Could you check a few things on this model? Use its own coordinates, in mm. Give positions to 0.01 mm unless a question says otherwise; leave off trailing zeros. Loops run counter-clockwise (first coordinate to the right, second up) from the corner with the lowest first, then second, coordinate; pieces in that order, holes last. Notation, with made-up numbers: (-29, 67) -> (-9, 67) arc R23 ccw to (-9, 78) -> close; hole circle Ø1 at (45.25, 41.5). An arc over 180 degrees is marked (long way). Write each question's results on one line, items separated by ' | '. Start each with the question number.
Q1. If we section it at A-A, the plane x = 32: List the corners of the cut face in (y, z) for me.
Q2. If we section it at D-D, the plane x = -97.5: List the corners of the cut face in (y, z) for me.
Q3. If we section it at B-B, the plane y = 51: List the corners of the cut face in (x, z) for me, plus the area to 3 significant figures.
Q4. If we section it at C-C, the plane z = 1: Give the number of separate pieces and of enclosed holes in the cut face, plus the area to 3 significant figures.
Q5. If I drill on line 1 along Y through (x, z) = (-14, 1.4); line 2 along X through (y, z) = (64, 0.85); line 3 along X through (y, z) = (10.5, 1.15), over which ranges is the centre line in solid material (lowest first)?
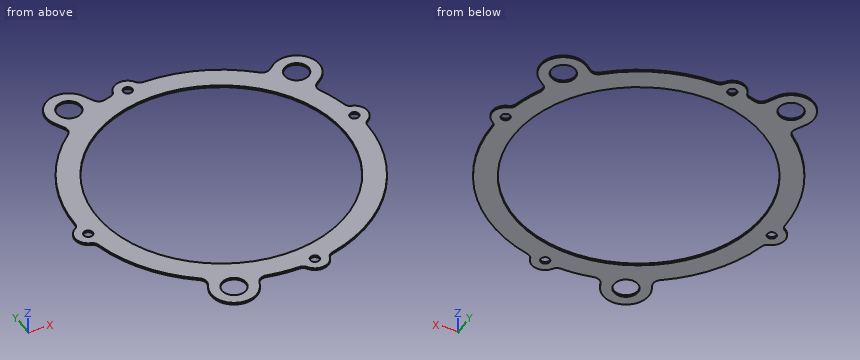
from build123d import *

# Parameters (mm, degrees)
F0_R     = 9
F0_R_2   = 3.4
F0_R_3   = 92.5
F1_DEPTH = 1.5
F2_R     = 6
F3_R     = 5


# Not quite as in the source:
# - a feature names something its author has since deleted; it is built from what else it names


with BuildPart() as f1:
    # F0 (on Top) → F1 (new body)
    with BuildSketch(Plane.XY):
        with BuildLine():
            ThreePointArc((-41.5612142371, 114.3762015069), (-64.5523398831, 121.4052940181), (-71.5814323943, 98.4141683721))
            Line((-71.5814323943, 98.4141683721), (-65.4484708904, 86.8797453608))
            ThreePointArc((-65.4484708904, 86.8797453608), (-98.0871820311, 47.0159251428), (-108.7201014418, -3.3958854983))
            ThreePointArc((-108.7201014418, -3.3958854983), (-115.9027148008, -14.2310639443), (-106.3121888463, -23.0067598447))
            ThreePointArc((-106.3121888463, -23.0067598447), (-89.5246549559, -61.7812969341), (-59.2286170286, -91.2335652089))
            Line((-59.2286170286, -91.2335652089), (-62.9150916983, -99.5135228831))
            ThreePointArc((-62.9150916983, -99.5135228831), (-54.2993418506, -121.9583185953), (-31.8545461384, -113.3425687477))
            Line((-31.8545461384, -113.3425687477), (-28.1680714687, -105.0626110734))
            ThreePointArc((-28.1680714687, -105.0626110734), (-12.5203677417, -108.0501406174), (3.3958854983, -108.7201014418))
            ThreePointArc((3.3958854983, -108.7201014418), (14.2310639443, -115.9027148008), (23.0067598447, -106.3121888463))
            ThreePointArc((23.0067598447, -106.3121888463), (85.7143913832, -66.9674219725), (108.7201014418, 3.3958854983))
            ThreePointArc((108.7201014418, 3.3958854983), (115.9027148008, 14.2310639443), (106.3121888463, 23.0067598447))
            ThreePointArc((106.3121888463, 23.0067598447), (102.1418848281, 37.3982333755), (96.0334257824, 51.0800707549))
            Line((96.0334257824, 51.0800707549), (104.0705278241, 57.1364615496))
            ThreePointArc((104.0705278241, 57.1364615496), (107.4164761014, 80.944120614), (83.608817037, 84.2900688912))
            Line((83.608817037, 84.2900688912), (75.5717149953, 78.2336780965))
            ThreePointArc((75.5717149953, 78.2336780965), (39.1751591317, 101.4736389554), (-3.3958854983, 108.7201014418))
            ThreePointArc((-3.3958854983, 108.7201014418), (-14.2310639443, 115.9027148008), (-23.0067598447, 106.3121888463))
            ThreePointArc((-23.0067598447, 106.3121888463), (-29.2689871835, 104.7612470577), (-35.4282527332, 102.8417784955))
            Line((-35.4282527332, 102.8417784955), (-41.5612142371, 114.3762015069))
        make_face()
        with Locations((-47.3848189183, -106.4280458154)):
            Circle(F0_R, mode=Mode.SUBTRACT)
        with Locations((-105.9772532844, -13.0123705102)):
            Circle(F0_R_2, mode=Mode.SUBTRACT)
        with Locations((13.0123705102, -105.9772532844)):
            Circle(F0_R_2, mode=Mode.SUBTRACT)
        Circle(F0_R_3, mode=Mode.SUBTRACT)
        with Locations((-56.5713233157, 106.3951849395)):
            Circle(F0_R, mode=Mode.SUBTRACT)
        with Locations((-13.0123705102, 105.9772532844)):
            Circle(F0_R_2, mode=Mode.SUBTRACT)
        with Locations((105.9772532844, 13.0123705102)):
            Circle(F0_R_2, mode=Mode.SUBTRACT)
        with Locations((93.8396724306, 70.7132652204)):
            Circle(F0_R, mode=Mode.SUBTRACT)
    extrude(amount=F1_DEPTH)

    # F2
    f2_edges = [f1.edges().sort_by_distance(p)[0] for p in [
        (-65.448471, 86.879745, 0.75),
        (-59.228617, -91.233565, 0.75),
        (-28.168071, -105.062611, 0.75),
        (96.033426, 51.080071, 0.75),
        (75.571715, 78.233678, 0.75),
        (-35.428253, 102.841778, 0.75),
    ]]
    fillet(f2_edges, radius=F2_R)

    # F3
    f3_edges = [f1.edges().sort_by_distance(p)[0] for p in [
        (-108.720101, -3.395885, 0.75),
        (-106.312189, -23.00676, 0.75),
        (-23.00676, 106.312189, 0.75),
        (-3.395885, 108.720101, 0.75),
        (3.395885, -108.720101, 0.75),
        (23.00676, -106.312189, 0.75),
        (108.720101, 3.395885, 0.75),
        (106.312189, 23.00676, 0.75),
    ]]
    fillet(f3_edges, radius=F3_R)


solid = f1.part
Final values:
1) outline: (-103.96, 0) -> (-86.79, 0) -> (-86.79, 1.5) -> (-103.96, 1.5) -> close; (86.79, 0) -> (103.96, 0) -> (103.96, 1.5) -> (86.79, 1.5) -> close
2) outline: (-48.22, 0) -> (48.22, 0) -> (48.22, 1.5) -> (-48.22, 1.5) -> close
3) outline: (-96.08, 0) -> (-77.17, 0) -> (-77.17, 1.5) -> (-96.08, 1.5) -> close; (77.17, 0) -> (97.89, 0) -> (97.89, 1.5) -> (77.17, 1.5) -> close | area: 59.4 mm²
4) separate pieces: 1 | enclosed holes: 8 | area: 12,300 mm²
5) line 1: y = -107.87 to -91.43, 91.43 to 102.72, 109.23 to 115.93 | line 2: x = -87.95 to -66.79, 66.79 to 87.85, 99.83 to 109.46 | line 3: x = -108.27 to -91.9, 91.9 to 103.69, 108.27 to 115.66
